```python
from build123d import *

# Parameters (mm, degrees)
SKETCH1_W              = 482.6
SKETCH1_H              = 265.938
BOSS_EXTRUDE1_DEPTH    = 3.175
CUT_EXTRUDE1_DEPTH     = 4.175
CUT_EXTRUDE2_DEPTH     = 4.175
SKETCH4_R              = 4.7625
CUT_EXTRUDE3_DEPTH     = 4.175
SKETCH5_R              = 4.7625
CUT_EXTRUDE4_DEPTH     = 4.175
F_4_CLEARANCE_HOLE1_D  = 3.2639
SKETCH8_R              = 5
SKETCH8_R_2            = 3.175
SKETCH8_R_3            = 6.35
CUT_EXTRUDE5_DEPTH     = 4.175
SKETCH9_R              = 4.7625
CUT_EXTRUDE6_DEPTH     = 4.175
SKETCH10_R             = 3.175
SKETCH10_R_2           = 4.7625
CUT_EXTRUDE7_DEPTH     = 4.175
F_6_32_TAPPED_HOLE_D   = 2.7051
F_10_32_TAPPED_HOLE1_D = 4.0386
SKETCH15_R             = 4.7625
CUT_EXTRUDE8_DEPTH     = 4.175
SKETCH16_R             = 4.7625
CUT_EXTRUDE9_DEPTH     = 4.175
F_10_CLEARANCE_HOLE1_D = 5.1054


with BuildPart() as part:
    # Sketch1 → Boss-Extrude1 (new body)
    with BuildSketch(Plane.XY):
        Rectangle(SKETCH1_W, SKETCH1_H)
    extrude(amount=BOSS_EXTRUDE1_DEPTH)

    # Sketch2 → Cut-Extrude1 (cut, through all)
    with BuildSketch(Plane.XY.offset(3.175)):
        with BuildLine():
            Line((-234.442, 98.806), (-231.14, 98.806))
            ThreePointArc((-231.14, 98.806), (-227.584, 95.25), (-231.14, 91.694))
            Line((-231.14, 91.694), (-234.442, 91.694))
            ThreePointArc((-234.442, 91.694), (-237.998, 95.25), (-234.442, 98.806))
        make_face()
        with BuildLine():
            Line((-234.442, 41.656), (-231.14, 41.656))
            ThreePointArc((-231.14, 41.656), (-227.584, 38.1), (-231.14, 34.544))
            Line((-231.14, 34.544), (-234.442, 34.544))
            ThreePointArc((-234.442, 34.544), (-237.998, 38.1), (-234.442, 41.656))
        make_face()
        with BuildLine():
            Line((-234.442, -34.544), (-231.14, -34.544))
            ThreePointArc((-231.14, -34.544), (-227.584, -38.1), (-231.14, -41.656))
            Line((-231.14, -41.656), (-234.442, -41.656))
            ThreePointArc((-234.442, -41.656), (-237.998, -38.1), (-234.442, -34.544))
        make_face()
        with BuildLine():
            Line((-234.442, -91.694), (-231.14, -91.694))
            ThreePointArc((-231.14, -91.694), (-227.584, -95.25), (-231.14, -98.806))
            Line((-231.14, -98.806), (-234.442, -98.806))
            ThreePointArc((-234.442, -98.806), (-237.998, -95.25), (-234.442, -91.694))
        make_face()
    cut_extrude1 = extrude(amount=-CUT_EXTRUDE1_DEPTH, mode=Mode.SUBTRACT)

    # Mirror1: Cut-Extrude1 across plane
    add(cut_extrude1.mirror(Plane(origin=(0, 0, 0), x_dir=(0, 0, 1), z_dir=(1, 0, 0))), mode=Mode.SUBTRACT)

    # Sketch3 → Cut-Extrude2 (cut, through all)
    with BuildSketch(Plane(origin=(-181.02162033, -243.631772018, 3.175), x_dir=(1, 0, 0), z_dir=(0, 0, 1))):
        with BuildLine():
            Line((181.048825452, 369.772362154), (181.048825452, 364.379181883))
            ThreePointArc((181.048825452, 364.379181883), (177.873825452, 362.910172018), (174.698825452, 364.379181883))
            Line((174.698825452, 364.379181883), (174.698825452, 369.772362154))
            ThreePointArc((174.698825452, 369.772362154), (177.873825452, 371.241372018), (181.048825452, 369.772362154))
        make_face()
        with BuildLine():
            Line((161.998825452, 369.772362154), (161.998825452, 364.379181883))
            ThreePointArc((161.998825452, 364.379181883), (158.823825452, 362.910172018), (155.648825452, 364.379181883))
            Line((155.648825452, 364.379181883), (155.648825452, 369.772362154))
            ThreePointArc((155.648825452, 369.772362154), (158.823825452, 371.241372018), (161.998825452, 369.772362154))
        make_face()
        with BuildLine():
            Line((161.998825452, 357.072362154), (161.998825452, 351.679181883))
            ThreePointArc((161.998825452, 351.679181883), (158.823825452, 350.210172018), (155.648825452, 351.679181883))
            Line((155.648825452, 351.679181883), (155.648825452, 357.072362154))
            ThreePointArc((155.648825452, 357.072362154), (158.823825452, 358.541372018), (161.998825452, 357.072362154))
        make_face()
        with BuildLine():
            Line((174.698825452, 357.072362154), (174.698825452, 351.679181883))
            ThreePointArc((174.698825452, 351.679181883), (177.873825452, 350.210172018), (181.048825452, 351.679181883))
            Line((181.048825452, 351.679181883), (181.048825452, 357.072362154))
            ThreePointArc((181.048825452, 357.072362154), (177.873825452, 358.541372018), (174.698825452, 357.072362154))
        make_face()
    extrude(amount=-CUT_EXTRUDE2_DEPTH, mode=Mode.SUBTRACT)

    # Sketch4 → Cut-Extrude3 (cut, through all)
    with BuildSketch(Plane(origin=(-181.02162033, -243.631772018, 3.175), x_dir=(1, 0, 0), z_dir=(0, 0, 1))):
        with Locations((97.88742033, 360.651377141)):
            Circle(SKETCH4_R)
        with Locations((36.946803704, 360.651377141)):
            Circle(SKETCH4_R)
    extrude(amount=-CUT_EXTRUDE3_DEPTH, mode=Mode.SUBTRACT)

    # Sketch5 → Cut-Extrude4 (cut, through all)
    with BuildSketch(Plane(origin=(-181.02162033, -243.631772018, 3.175), x_dir=(1, 0, 0), z_dir=(0, 0, 1))):
        with Locations((225.993210145, 348.025772018)):
            Circle(SKETCH5_R)
        with Locations((292.693482391, 161.058252354)):
            Circle(SKETCH5_R)
    extrude(amount=-CUT_EXTRUDE4_DEPTH, mode=Mode.SUBTRACT)

    # #4 Clearance Hole1 (through all)
    with Locations(Plane(origin=(-181.02162033, -243.631772018, 0), x_dir=(-1, 0, 0), z_dir=(0, 0, -1))):
        with Locations((-127.09742033, 343.110872018), (-25.49742033, 343.110872018), (-25.49742033, 216.110872018), (-127.09742033, 216.110872018)):
            Hole(F_4_CLEARANCE_HOLE1_D / 2)

    # Sketch8 → Cut-Extrude5 (cut, through all)
    with BuildSketch(Plane(origin=(-181.02162033, -243.631772018, 3.175), x_dir=(1, 0, 0), z_dir=(0, 0, 1))):
        with Locations((87.210707903, 183.695733345)):
            Circle(SKETCH8_R)
        with Locations((103.085707903, 183.695733345)):
            Circle(SKETCH8_R)
        with Locations((118.960707903, 183.695733345)):
            Circle(SKETCH8_R)
        with Locations((134.835707903, 183.695733345)):
            Circle(SKETCH8_R)
        with Locations((134.835707903, 167.820733345)):
            Circle(SKETCH8_R)
        with Locations((118.960707903, 167.820733345)):
            Circle(SKETCH8_R)
        with Locations((103.085707903, 167.820733345)):
            Circle(SKETCH8_R)
        with Locations((87.210707903, 167.820733345)):
            Circle(SKETCH8_R)
        with Locations((71.335707903, 188.458233345)):
            Circle(SKETCH8_R_2)
        with Locations((71.335707903, 163.058233345)):
            Circle(SKETCH8_R_2)
        with Locations((103.085707903, 136.070733345)):
            Circle(SKETCH8_R_3)
        with Locations((134.835707903, 136.070733345)):
            Circle(SKETCH8_R_3)
        with Locations((77.685707903, 136.070733345)):
            Circle(SKETCH8_R_2)
    extrude(amount=-CUT_EXTRUDE5_DEPTH, mode=Mode.SUBTRACT)

    # Sketch9 → Cut-Extrude6 (cut, through all)
    with BuildSketch(Plane(origin=(-181.02162033, -243.631772018, 3.175), x_dir=(1, 0, 0), z_dir=(0, 0, 1))):
        with Locations((26.393194264, 192.958772018)):
            Circle(SKETCH9_R)
        with Locations((1.630666307, 192.958772018)):
            Circle(SKETCH9_R)
        with Locations((1.630666307, 123.362772018)):
            Circle(SKETCH9_R)
        with Locations((26.393194264, 123.362772018)):
            Circle(SKETCH9_R)
        with Locations((-27.185282018, 164.860944472)):
            Circle(SKETCH9_R)
    extrude(amount=-CUT_EXTRUDE6_DEPTH, mode=Mode.SUBTRACT)

    # Sketch10 → Cut-Extrude7 (cut, through all)
    with BuildSketch(Plane(origin=(-181.02162033, -243.631772018, 3.175), x_dir=(1, 0, 0), z_dir=(0, 0, 1))):
        with Locations((-15.753984793, 312.422144018)):
            Circle(SKETCH10_R)
        with Locations((-6.228984793, 331.472144018)):
            Circle(SKETCH10_R_2)
    extrude(amount=-CUT_EXTRUDE7_DEPTH, mode=Mode.SUBTRACT)

    # #6-32 Tapped Hole (through all)
    with Locations(Plane(origin=(-181.02162033, -243.631772018, 3.175), x_dir=(1, 0, 0), z_dir=(0, 0, 1))):
        with Locations((-13.634382018, 182.582872018), (47.401817982, 182.582872018), (47.401817982, 133.738672018), (-13.634382018, 133.738672018), (332.15162033, 353.232772018), (379.90362033, 353.232772018), (379.90362033, 310.179772018), (332.153973797, 310.179772018)):
            Hole(F_6_32_TAPPED_HOLE_D / 2)

    # #10-32 Tapped Hole1 (through all)
    with Locations(Plane(origin=(-181.02162033, -243.631772018, 3.175), x_dir=(1, 0, 0), z_dir=(0, 0, 1))):
        with Locations((278.168010145, 333.298282981), (173.774010145, 333.298282981), (173.774010145, 151.027882981), (278.168010145, 151.027882981)):
            Hole(F_10_32_TAPPED_HOLE1_D / 2)

    # Sketch15 → Cut-Extrude8 (cut, through all)
    with BuildSketch(Plane(origin=(-181.02162033, -243.631772018, 3.175), x_dir=(1, 0, 0), z_dir=(0, 0, 1))):
        with Locations((321.48362033, 331.756823693)):
            Circle(SKETCH15_R)
        with Locations((356.032924126, 363.900772018)):
            Circle(SKETCH15_R)
        with Locations((390.57162033, 331.759308089)):
            Circle(SKETCH15_R)
    extrude(amount=-CUT_EXTRUDE8_DEPTH, mode=Mode.SUBTRACT)

    # Sketch16 → Cut-Extrude9 (cut, through all)
    with BuildSketch(Plane(origin=(-181.02162033, -243.631772018, 3.175), x_dir=(1, 0, 0), z_dir=(0, 0, 1))):
        with Locations((335.161382997, 182.894837455)):
            Circle(SKETCH16_R)
        with Locations((348.023271542, 182.894837455)):
            Circle(SKETCH16_R)
    extrude(amount=-CUT_EXTRUDE9_DEPTH, mode=Mode.SUBTRACT)

    # #10 Clearance Hole1 (through all)
    with Locations(Plane(origin=(-181.02162033, -243.631772018, 3.175), x_dir=(1, 0, 0), z_dir=(0, 0, 1))):
        with Locations((-22.17837967, 363.900772018), (384.22162033, 363.900772018), (384.22162033, 123.362772018), (-22.17837967, 123.362772018)):
            Hole(F_10_CLEARANCE_HOLE1_D / 2)


solid = part.part
```
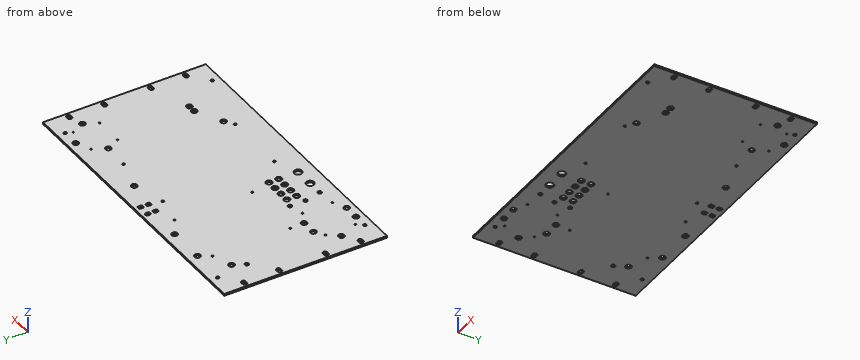
Design review of the part built by this model. Coordinates are the model's own, in mm. Give positions to 0.01 mm unless a question says otherwise; leave off trailing zeros. Write each loop counter-clockwise with the first axis right and the second up, starting at its lowest first coordinate (ties: lowest second). Pieces come first, ordered by that corner, then holes.
(1) Add section A-A (x = 112). Give the boundary of the cut face in (y, z) (3 decimals), and give its area (3 significant figures).
Checked values:
outline: (-132.969, 0) - (-87.325, 0) - (-87.325, 3.175) - (-132.969, 3.175) - close; (-77.822, 0) - (132.969, 0) - (132.969, 3.175) - (-77.822, 3.175) - close
area: 814 mm2
(2) Wall thickness on line 1 along Y through (x, z) = (-179, 2.25); line 2 along Y through (x, z) = (112, 2.95); line 3 along X through (y, z) = (-108.5, 0.65): over which ranges is each line inside the solid? List them lowest first.
Checked values:
line 1: y = -132.97 to -125.02, -115.52 to -55.42, -45.93 to 132.97
line 2: y = -132.97 to -87.32, -77.82 to 132.97
line 3: x = -241.3 to -106.37, -100.3 to -84.22, -71.66 to -52.47, -39.91 to 241.3
(3) Clearance check with flat-ended pins moving along their axes: pin 1 Ø10 at (x, y) = (-122, -94.5) entering from -Z; pin 2 Ø7.5 at (x, y) = (111.67, -82.57) entering from +Z. State where each tip first meets the part, or that it passes through.
Checked values:
pin 1: stops at z = 0
pin 2: passes through
